Here's how the part is built. I have some questions about the finished solid (model axes, mm). Round coordinates to 2 decimals unless told otherwise and drop trailing zeros. Write each loop counter-clockwise with the first axis right and the second up, starting at its lowest first coordinate (ties: lowest second). Pieces come first, ordered by that corner, then holes. Notation, with made-up numbers: (-27, 69.5) -> (18, 69.5) arc R19 ccw to (18, 73.5) -> close; hole circle Ø2 at (-33, 81.25). An arc over 180 degrees is marked (long way). Answer as CSV lines item,"result".
```python
from build123d import *

# Parameters (mm, degrees)
SKETCH_1_R      = 60
SKETCH_1_R_2    = 2.55
EXTRUDE_1_DEPTH = 4
CHAMFER_1_SIZE  = 2.5


with BuildPart() as part:
    # 草图1 → 凸台-拉伸1 (new body)
    with BuildSketch(Plane(origin=(0, 0, 0), x_dir=(1, 0, 0), z_dir=(0, 1, 0))):
        Circle(SKETCH_1_R)
        with Locations((0, 50)):
            Circle(SKETCH_1_R_2, mode=Mode.SUBTRACT)
        with Locations((50, 0)):
            Circle(SKETCH_1_R_2, mode=Mode.SUBTRACT)
        with Locations((0, -50)):
            Circle(SKETCH_1_R_2, mode=Mode.SUBTRACT)
        with Locations((-50, 0)):
            Circle(SKETCH_1_R_2, mode=Mode.SUBTRACT)
        with Locations((0, 40)):
            Circle(SKETCH_1_R_2, mode=Mode.SUBTRACT)
        with Locations((40, 0)):
            Circle(SKETCH_1_R_2, mode=Mode.SUBTRACT)
        with Locations((0, -40)):
            Circle(SKETCH_1_R_2, mode=Mode.SUBTRACT)
        with Locations((-40, 0)):
            Circle(SKETCH_1_R_2, mode=Mode.SUBTRACT)
        with Locations((0, 23)):
            Circle(SKETCH_1_R_2, mode=Mode.SUBTRACT)
        with Locations((23, 0)):
            Circle(SKETCH_1_R_2, mode=Mode.SUBTRACT)
        with Locations((0, -23)):
            Circle(SKETCH_1_R_2, mode=Mode.SUBTRACT)
        with Locations((-23, 0)):
            Circle(SKETCH_1_R_2, mode=Mode.SUBTRACT)
    extrude(amount=EXTRUDE_1_DEPTH)

    # 倒角1
    chamfer_1_edges = [part.edges().sort_by_distance(p)[0] for p in [
        (-2.55, 0, -23),
        (20.45, 0, 0),
        (-2.55, 0, 23),
        (-25.55, 0, 0),
    ]]
    chamfer(chamfer_1_edges, length=CHAMFER_1_SIZE)


solid = part.part
```
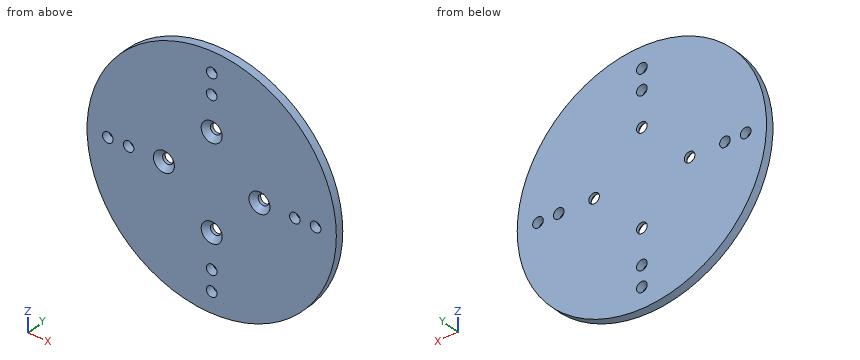
1. Suppose I cut it at A-A on y = 3.15. Count the separate pieces of the cut face and the enclosed holes in it, and give its area (3 significant figures).
Numbers:
separate pieces,"1"
enclosed holes,"12"
area,"11,100 mm^2"
2. Suppose I cut it at C-C on x = -23. Please give me the cut outline in (y, z), and give its area (3 significant figures).
Numbers:
outline,"(0, -55.42) -> (4, -55.42) -> (4, -2.55) -> (2.5, -2.55) -> (0, -5.05) -> close; (0, 5.05) -> (2.5, 2.55) -> (4, 2.55) -> (4, 55.42) -> (0, 55.42) -> close"
area,"417 mm^2"
3. If I drill on line 1 (Z direction, x = -40, y = 2.7); line 2 (X direction, y = 3.25, z = 23), over which ranges is the centre line in solid material (lowest first)?
Numbers:
line 1,"z = -44.72 to -2.55, 2.55 to 44.72"
line 2,"x = -55.42 to -2.55, 2.55 to 55.42"
4. For pin 1 Ø1.5 at (y, z) = (1, 24) entering from +X; pin 2 Ø2 at (y, z) = (2.5, 26.5) entering from +X; pin 3 Ø2 at (x, y) = (29, 2.5) entering from -Z, each with a flat end and sliding along its axis, tell me the tip position at first contact or that it passes through.
Numbers:
pin 1,"stops at x = 55.31"
pin 2,"stops at x = 54.31"
pin 3,"stops at z = -53.07"
5. Suppose I cut it at B-B on z = -23. Please give me the cut outline in (x, y).
Numbers:
outline,"(-55.42, 0) -> (-5.05, 0) -> (-2.55, 2.5) -> (-2.55, 4) -> (-55.42, 4) -> close; (2.55, 2.5) -> (5.05, 0) -> (55.42, 0) -> (55.42, 4) -> (2.55, 4) -> close"
6. Suppose I cut it at D-D on z = -40. Please give me the cut outline in (x, y), and give its area (3 significant figures).
Numbers:
outline,"(-44.72, 0) -> (-2.55, 0) -> (-2.55, 4) -> (-44.72, 4) -> close; (2.55, 0) -> (44.72, 0) -> (44.72, 4) -> (2.55, 4) -> close"
area,"337 mm^2"
